Read the model definition and answer for the solid it produces. Units are mm, in the model's axes. Face numbers are marked on the shaded views. A direction names the side the tool comes from. Coordinates: 2 decimals unless noted, no trailing zeros. Loops run counter-clockwise (first coordinate to the right, second up) from the corner with the lowest first, then second, coordinate; pieces in that order, holes last. Notation, with made-up numbers: M -12.75,25 L 41.25,25 A14 ccw 41.25,48 Z; hole C 27.5,62 d7. An arc over 180 degrees is marked long. Put each result on its own line as item: value.
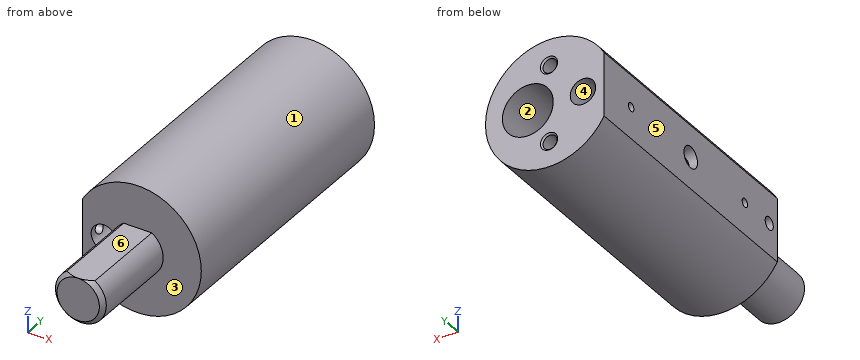
from build123d import *

# Parameters (mm, degrees)
BOSS_EXTRUDE1_DEPTH         = 22
BOSS_EXTRUDE2_DEPTH         = 64
SKETCH3_R                   = 3
CUT_EXTRUDE1_DEPTH          = 65
SKETCH4_R                   = 6
CUT_EXTRUDE2_DEPTH          = 52
M4_TAPPED_HOLE1_D           = 3.3
M4_TAPPED_HOLE1_DEPTH       = 14
M4_TAPPED_HOLE1_CSINK_D     = 4.05
M4_TAPPED_HOLE1_CSINK_ANGLE = 90
M4_TAPPED_HOLE1_TIP         = 0.991420021
SKETCH7_R                   = 2.5
SKETCH7_R_2                 = 1.5
CUT_EXTRUDE3_DEPTH          = 5
SKETCH8_R                   = 1
CUT_EXTRUDE4_DEPTH          = 15
CHAMFER1_SIZE               = 1


with BuildPart() as part:
    # Sketch1 → Boss-Extrude1 (new body)
    with BuildSketch(Plane(origin=(0, 0, 0), x_dir=(1, 0, 0), z_dir=(0, 1, 0))):
        with BuildLine():
            Line((-3.31662479, -5), (3.31662479, -5))
            ThreePointArc((3.31662479, -5), (0, 6), (-3.31662479, -5))
        make_face()
    extrude(amount=BOSS_EXTRUDE1_DEPTH)

    # Sketch2 → Boss-Extrude2 (add)
    with BuildSketch(Plane(origin=(0, 22, 0), x_dir=(1, 0, 0), z_dir=(0, 1, 0))):
        with BuildLine():
            Line((-13, 7.483314774), (-13, -7.483314774))
            ThreePointArc((-13, -7.483314774), (15, 0), (-13, 7.483314774))
        make_face()
    extrude(amount=BOSS_EXTRUDE2_DEPTH)

    # Sketch3 → Cut-Extrude1 (cut)
    with BuildSketch(Plane(origin=(0, 86, 0), x_dir=(1, 0, 0), z_dir=(0, 1, 0))):
        with Locations(Location((-8, 0, 0), (0, 0, 270))):
            Circle(SKETCH3_R)
    extrude(amount=-CUT_EXTRUDE1_DEPTH, mode=Mode.SUBTRACT)

    # Sketch4 → Cut-Extrude2 (cut)
    with BuildSketch(Plane(origin=(0, 86, 0), x_dir=(1, 0, 0), z_dir=(0, 1, 0))):
        with Locations(Location((5, 0, 0), (0, 0, 270))):
            Circle(SKETCH4_R)
    extrude(amount=-CUT_EXTRUDE2_DEPTH, mode=Mode.SUBTRACT)

    # M4 Tapped Hole1
    with Locations(Plane(origin=(0, 86, 0), x_dir=(1, 0, 0), z_dir=(0, 1, 0))):
        with Locations((0, 9), (0, -9)):
            CounterSinkHole(M4_TAPPED_HOLE1_D / 2, M4_TAPPED_HOLE1_CSINK_D / 2, depth=M4_TAPPED_HOLE1_DEPTH, counter_sink_angle=M4_TAPPED_HOLE1_CSINK_ANGLE)
            with Locations((0, 0, -(M4_TAPPED_HOLE1_DEPTH + M4_TAPPED_HOLE1_TIP / 2))):  # 118° drill point
                Cone(0, M4_TAPPED_HOLE1_D / 2, M4_TAPPED_HOLE1_TIP, mode=Mode.SUBTRACT)

    # Sketch7 → Cut-Extrude3 (cut)
    with BuildSketch(Plane.ZY.offset(13)):
        with Locations((0, 54)):
            Circle(SKETCH7_R)
        with Locations((0, 25)):
            Circle(SKETCH7_R_2)
    extrude(amount=-CUT_EXTRUDE3_DEPTH, mode=Mode.SUBTRACT)

    # Sketch8 → Cut-Extrude4 (cut)
    with BuildSketch(Plane.ZY.offset(13)):
        with Locations((0, 76)):
            Circle(SKETCH8_R)
        with Locations((0, 34)):
            Circle(SKETCH8_R)
    extrude(amount=-CUT_EXTRUDE4_DEPTH, mode=Mode.SUBTRACT)

    # Chamfer1
    chamfer1_edges = [part.edges().sort_by_distance(p)[0] for p in [
        (0, 0, -6),
    ]]
    chamfer(chamfer1_edges, length=CHAMFER1_SIZE - 0.0001)  # a hair under: the kernel refuses the full size


solid = part.part
1) Find section D-D, the plane y = 10. Write down the section's boundary in (x, z), plus the area to 3 significant figures.
Answer list:
outline: M -3.32,5 A6 ccw long 3.32,5 Z
area: 109 mm^2
2) Determine the mould class of the marked faces 4, 5 and 6 for opening direction Z: released by +Z, released by -Z, zero draft, split by the parting line, or undercut.
Answer list:
face 4: undercut
face 5: zero draft
face 6: released by +Z
3) Find section A-A, the plane y = 76. Write down the section's boundary in (x, z).
Answer list:
outline: M -13,-7.48 A15 ccw long -13,7.48 L -13,1 L -10.83,1 A3 cw -5.17,1 L -0.92,1 A6 cw long -0.92,-1 L -5.17,-1 A3 cw -10.83,-1 L -13,-1 Z; hole C 0,-9 d3.3; hole C 0,9 d3.3
4) Given pin 1 Ø8 at (x, y) = (-8, 47.5) entering from -Z; pin 2 Ø2 at (x, y) = (10, 67.5) entering from +Z; pin 3 Ø7 at (x, z) = (5, 0) entering from +Y, each flat-ended and moving along its own axis, determine where each tip first touches the part or whether it passes through.
Answer list:
pin 1: stops at z = -14.46
pin 2: stops at z = 12
pin 3: stops at y = 34
5) Straight lines are drawn through the part: line 1 (X direction, y = 68.5, z = 0); line 2 (X direction, y = 56, z = 0); line 3 (Y direction, x = -4.25, z = 11). For each, find the intervals that lie inside material, in ascending order. Write a range as [from, to].
Answer list:
line 1: x = [-13, -11], [-5, -1], [11, 15]
line 2: x = [-5, -1], [11, 15]
line 3: y = [22, 86]
6) Which of the six approach directions +Z, -Z, +X, -X, +Y, -Y give full straight-line access (tool end or side, diameter ignored) to the marked faces 1, 2 and 3?
Answer list:
face 1: +Y, -Y
face 2: +Y
face 3: -Y
7) Find section B-B, the plane x = 9.75. Write down the section's boundary in (y, z).
Answer list:
outline: M 22,-11.4 L 86,-11.4 L 86,-3.67 L 34,-3.67 L 34,3.67 L 86,3.67 L 86,11.4 L 22,11.4 Z
8) Find section C-C, the plane y = 29. Write down the section's boundary in (x, z).
Answer list:
outline: M -13,-7.48 A15 ccw long -13,7.48 Z; hole C -8,0 d6
